Check sheet for the drawn part. Datum: minimum x, y, z corner. Units: mm. A direction names the side the tool comes from. Give positions to 0.01 mm unless a question says otherwise; leave off trailing zeros. Order: outer loops, then holes, each group sorted by start corner. A loop starts at its lowest first (then second) coordinate and runs counter-clockwise, first axis right, second up. Notation, with made-up numbers: (64, 2.25) -> (80, 2.25) arc R16 cw to (80, 31.25) -> close; hole circle Ø10 at (17, 55). An arc over 180 degrees is marked (long way). Answer in a Markdown table with one row per item. Add a question column.
(1) Go/stop test with flat-tipped pins: pin 1 (16 mm diameter, centred on x = 30, y = 35, fed in from +Z); pin 2 (12 mm diameter, centred on x = 78.5, y = 13, fed in from -Z); pin 3 (3 mm diameter, centred on y = 36.5, z = 28.5, fed in from +X); pin 4 (9 mm diameter, centred on x = 70, y = 25, fed in from -Z). Record where each tip stops, or that it passes through.
(2) Release check for a two-part mould opening along X. For the marked faces 4, 5 and 6 record: released by +X, released by -X, zero draft, split by the parting line, or undercut.
(3) Cross-section at B-B (z = 12.5). Record the cut outline in (x, y), then the cut area to 3 significant figures.
(4) Thickness scan on L1, parallel to Y at x = 30, z = 13; L2, parallel to Y at x = 70, z = 33.1; L3, parallel to Y at x = 27.5, z = 15. Record the ranges inside material, lowest first. Write a range as [from, to].
(5) Set-up check for the marked faces 1, 2 and 3: record each of +Z, -Z, +X, -X, +Y, -Y from which the full face is reachable in a straight line by a thin tool's end or side.
(6) Cross-section at C-C (y = 17). Record the cut outline in (x, z).
(7) Cross-section at A-A (x = 30). Record the cut outline in (y, z).
(8) Cross-section at D-D (x = 70). Record the cut outline in (y, z).
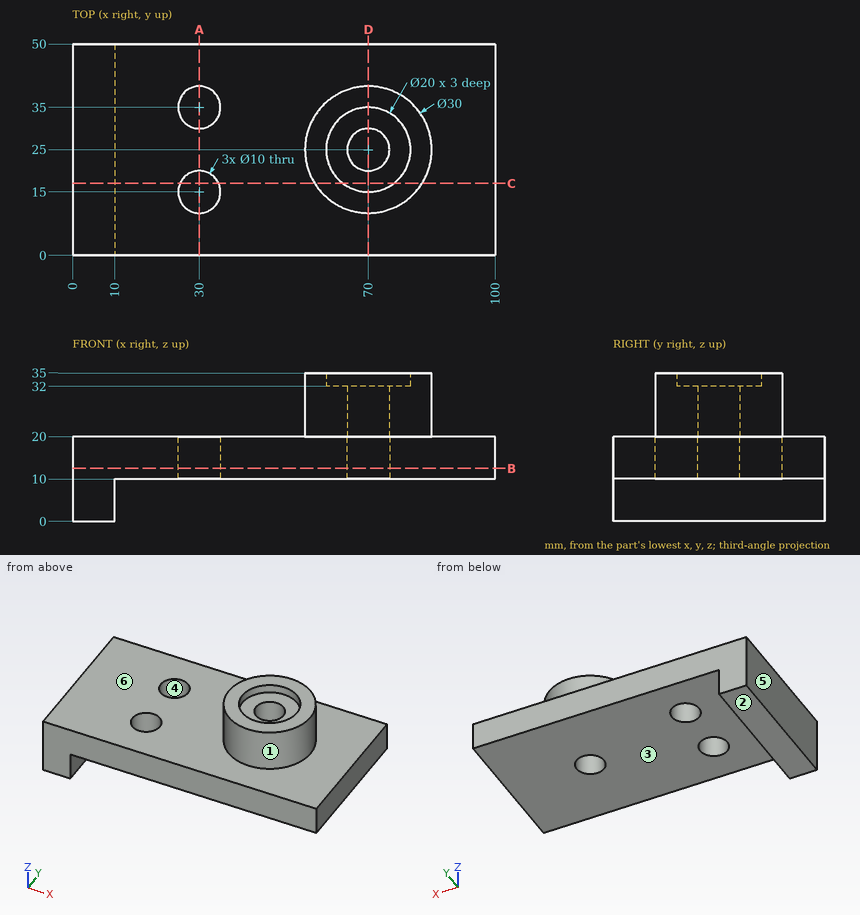
Answer below:
| question | item | result |
|---|---|---|
| 1 | pin 1 | stops at z = 20 |
| 1 | pin 2 | stops at z = 10 |
| 1 | pin 3 | stops at x = 81.18 |
| 1 | pin 4 | passes through |
| 2 | face 4 | undercut |
| 2 | face 5 | released by -X |
| 2 | face 6 | zero draft |
| 3 | outline | (0, 0) -> (100, 0) -> (100, 50) -> (0, 50) -> close; hole circle Ø10 at (30, 15); hole circle Ø10 at (30, 35); hole circle Ø10 at (70, 25) |
| 3 | area | 4,760 mm² |
| 4 | L1 | y = [0, 10], [20, 30], [40, 50] |
| 4 | L2 | y = [10, 15], [35, 40] |
| 4 | L3 | y = [0, 10.67], [19.33, 30.67], [39.33, 50] |
| 5 | face 1 | +Z |
| 5 | face 2 | -Z, +X, -X, +Y, -Y |
| 5 | face 3 | -Z, +X, +Y, -Y |
| 6 | outline | (0, 0) -> (10, 0) -> (10, 10) -> (25.42, 10) -> (25.42, 20) -> (0, 20) -> close; (34.58, 10) -> (100, 10) -> (100, 20) -> (82.69, 20) -> (82.69, 35) -> (76, 35) -> (76, 32) -> (64, 32) -> (64, 35) -> (57.31, 35) -> (57.31, 20) -> (34.58, 20) -> close |
| 7 | outline | (0, 10) -> (10, 10) -> (10, 20) -> (0, 20) -> close; (20, 10) -> (30, 10) -> (30, 20) -> (20, 20) -> close; (40, 10) -> (50, 10) -> (50, 20) -> (40, 20) -> close |
| 8 | outline | (0, 10) -> (20, 10) -> (20, 32) -> (15, 32) -> (15, 35) -> (10, 35) -> (10, 20) -> (0, 20) -> close; (30, 10) -> (50, 10) -> (50, 20) -> (40, 20) -> (40, 35) -> (35, 35) -> (35, 32) -> (30, 32) -> close |
